Design review of the part shown in the three views and the two pictorial views. Dimensions are in mm from the part's minimum x, y and z. Give positions to 0.01 mm unless a question says otherwise; leave off trailing zeros. Write each loop counter-clockwise with the first axis right and the second up, starting at its lowest first coordinate (ties: lowest second). Pieces come first, ordered by that corner, then holes. Notation, with made-up numbers: M -2.5,-8 L 13.5,-8 A13 ccw 13.5,1 Z; hole C 85.5,-15.5 d9. An arc over 180 degrees is marked long. Use one line per item in the form item = value. Start each with the question number.
Q1. For probe 1 along Z at (x, y) = (52.5, 4); probe 2 along Z at (x, y) = (205, 7.75); probe 3 along X at (y, z) = (9.5, 12.75), list the stretches that pass through material, from the lowest coordinate up. Write a range as [from, to].
Q2. Clearance check with a flat-ended pin moving along its axis: pin 1 Ø7.5 at (x, z) = (205, 10) entering from +Y. State where the tip first meets the part, or that it passes through.
Q3. Consider section B-B on x = 205. Write out the cut boundary in (y, z).
Q4. Consider section A-A on y = 10. Write out the cut boundary in (x, z), and give its area (3 significant figures).
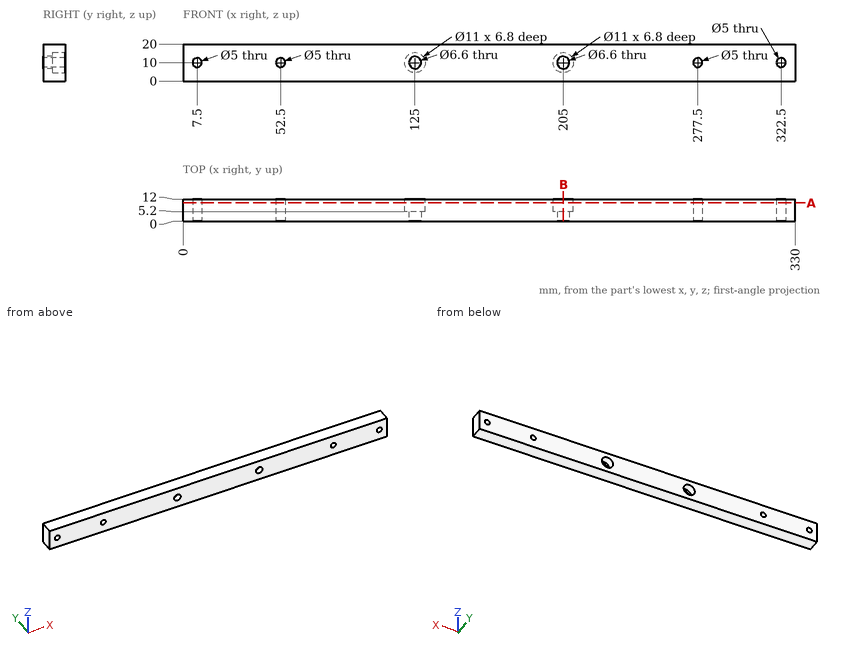
Working result:
q1.probe_1 = [0, 7.5], [12.5, 20]
q1.probe_2 = [0, 4.5], [15.5, 20]
q1.probe_3 = [0, 120.24], [129.76, 200.24], [209.76, 330]
q2.pin_1 = 5.2
q3.outline = M 0,0 L 12,0 L 12,4.5 L 5.2,4.5 L 5.2,6.7 L 0,6.7 Z; M 0,13.3 L 5.2,13.3 L 5.2,15.5 L 12,15.5 L 12,20 L 0,20 Z
q4.outline = M 0,0 L 330,0 L 330,20 L 0,20 Z; hole C 7.5,10 d5; hole C 52.5,10 d5; hole C 125,10 d11; hole C 205,10 d11; hole C 277.5,10 d5; hole C 322.5,10 d5
q4.area = 6,330 mm²
